Work out the finished part from the listing and answer in its coordinate system (mm). A direction names the side the tool comes from. Coordinates: 2 decimals unless noted, no trailing zeros. Write each loop counter-clockwise with the first axis right and the second up, starting at its lowest first coordinate (ties: lowest second). Pieces come first, ordered by that corner, then holes. Notation, with made-up numbers: (-2.5, 10) - (9.5, 10) arc R30 ccw to (9.5, 47) - close; hole circle Ø6 at (76.5, 8.25). An arc over 180 degrees is marked (long way). Use one line per item in the form item = value. Start each with the question number.
Item 1: A cutting plane is placed at B-B (x = 0). Write down the section's boundary in (y, z) (3 decimals).
Item 2: A cutting plane is placed at D-D (y = 8.25). Write down the section's boundary in (x, z) (3 decimals).
Item 3: A cutting plane is placed at C-C (z = 6). Write down the section's boundary in (x, y).
Item 4: A cutting plane is placed at A-A (z = 0). Write down the section's boundary in (x, y) (3 decimals).
Item 5: Determine the mould class of faces 3 (the flat face through (2.4, 20, -0.1)), 4 (the cylindrical face through (-9.76, 9.86, -2.17)), 5 (the flat face through (0, 10, 6)) for opening direction Z: released by +Z, released by -Z, zero draft, split by the parting line, or undercut.
Item 6: For faces 1 (the flat face through (2.4, 0, -0.1)), 2 (the flat face through (-5, 10, -3)), determine the directions among +Z, -Z, +X, -X, +Y, -Y from which every point of the face is accessible in a straight line to the end or side of a thin tool.
Item 7: Given pin 1 (2.5 mm diameter, centred on x = 0, z = 0, fed in from +Y); pin 2 (3 mm diameter, centred on x = 2, y = 11.5, fed in from -Z); pin 3 (1.5 mm diameter, centred on y = 12, z = 3.5, fed in from +X); pin 4 (1.5 mm diameter, centred on x = -5, z = -4, fed in from +Y), each flat-ended and moving along its own axis, determine where each tip first touches the part or whether it passes through.
Item 8: Consider probe 1 along X at (y, z) = (13.5, -4.5); probe 2 along X at (y, z) = (12.5, -3); probe 3 along X at (y, z) = (12.25, 0) (3 decimals). Determine where each line is inside the solid, lowest interval first.
from build123d import *

# Parameters (mm, degrees)
SKETCH1_R           = 10
BOSS_EXTRUDE1_DEPTH = 20
SKETCH2_R           = 2.5
CUT_EXTRUDE1_DEPTH  = 10
SKETCH2_3_R         = 2.125
CUT_EXTRUDE2_DEPTH  = 25.494897428


with BuildPart() as part:
    # Sketch1 → Boss-Extrude1 (new body)
    with BuildSketch(Plane(origin=(0, 0, 0), x_dir=(1, 0, 0), z_dir=(0, 1, 0))):
        with Locations(Location((0, 0, 0), (0, 0, 270))):
            Circle(SKETCH1_R)
    extrude(amount=BOSS_EXTRUDE1_DEPTH)

    # Sketch2 → Cut-Extrude1 (cut)
    with BuildSketch(Plane(origin=(0, 20, 0), x_dir=(1, 0, 0), z_dir=(0, 1, 0))):
        with Locations(Location((-5.196152423, 3, 0), (0, 0, 270))):
            Circle(SKETCH2_R)
        with Locations(Location((0, -6, 0), (0, 0, 270))):
            Circle(SKETCH2_R)
        with Locations(Location((5.196152423, 3, 0), (0, 0, 270))):
            Circle(SKETCH2_R)
    extrude(amount=-CUT_EXTRUDE1_DEPTH, mode=Mode.SUBTRACT)

    # Sketch2_3 → Cut-Extrude2 (cut, through all)
    with BuildSketch(Plane(origin=(0, 20, 0), x_dir=(1, 0, 0), z_dir=(0, 1, 0))):
        with Locations(Location((0, 0, 0), (0, 0, 270))):
            Circle(SKETCH2_3_R)
    extrude(amount=-CUT_EXTRUDE2_DEPTH, mode=Mode.SUBTRACT)


solid = part.part
Answer:
q1.outline = (0, -10) - (20, -10) - (20, -2.125) - (0, -2.125) - close; (0, 2.125) - (20, 2.125) - (20, 3.5) - (10, 3.5) - (10, 8.5) - (20, 8.5) - (20, 10) - (0, 10) - close
q2.outline = circle Ø20 at (0, 0); hole circle Ø4.25 at (0, 0)
q3.outline = (-8, 0) - (8, 0) - (8, 20) - (2.5, 20) - (2.5, 10) - (-2.5, 10) - (-2.5, 20) - (-8, 20) - close
q4.outline = (-10, 0) - (-2.125, 0) - (-2.125, 20) - (-10, 20) - close; (2.125, 0) - (10, 0) - (10, 20) - (2.125, 20) - close
q5.face_3 = zero draft
q5.face_4 = split by the parting line
q5.face_5 = undercut
q6.face_1 = +Z, -Z, +X, -X, -Y
q6.face_2 = +Y
q7.pin_1 = through
q7.pin_2 = -9.99
q7.pin_3 = 9.61
q7.pin_4 = 10
q8.probe_1 = -8.93 to -7.2, -3.2 to 3.2, 7.2 to 8.93
q8.probe_2 = -9.54 to -7.7, -2.7 to 2.7, 7.7 to 9.54
q8.probe_3 = -10 to -2.125, 2.125 to 10
